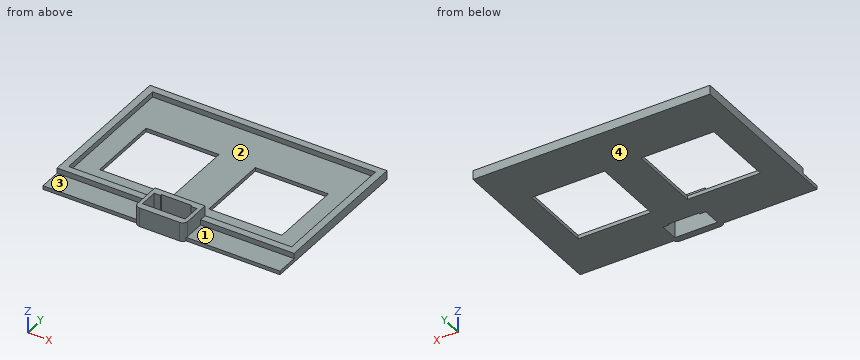
```python
from build123d import *

# Parameters (mm, degrees)
F0_W     = 38.1
F0_H     = 38.1
F1_DEPTH = 1.905
F0_W_2   = 48.74895
F0_H_2   = 11.557
F0_W_3   = 48.79975
F2_DEPTH = 4.699
F0_W_4   = 13.589
F0_H_3   = 3.5052
F3_DEPTH = 9.9314
F4_R     = 2.54


# Not quite as in the source:
# - a feature names something its author has since deleted; it is built from what else it names


with BuildPart() as f1:
    # F0 (on Top) → F1 (new body)
    with BuildSketch(Plane.XY):
        Polygon((-13.10005, -34.417), (13.04925, -34.417), (58.166, -34.417), (58.166, 34.417), (-58.166, 34.417), (-58.166, -34.417), align=None)
        with Locations((-28.5115, -6.604)):
            Rectangle(F0_W, F0_H, mode=Mode.SUBTRACT)
        with Locations((28.5115, -6.604)):
            Rectangle(F0_W, F0_H, mode=Mode.SUBTRACT)
    extrude(amount=F1_DEPTH)



with BuildPart() as f1b:
    # F0 (on Top) → F1, piece 2 (new body)
    with BuildSketch(Plane.XY):
        with Locations((-37.474525, -43.8785)):
            Rectangle(F0_W_2, F0_H_2)
    extrude(amount=F1_DEPTH)


with BuildPart() as f1c:
    # F0 (on Top) → F1, piece 3 (new body)
    with BuildSketch(Plane.XY):
        with Locations((37.449125, -43.8785)):
            Rectangle(F0_W_3, F0_H_2)
    extrude(amount=F1_DEPTH)


with BuildPart() as f1_1:
    add(f1.part)

    add(f1b.part)  # F2 merges F1b

    add(f1c.part)  # F2 merges F1c
    # F0 (on Top) → F2 (join)
    with BuildSketch(Plane.XY):
        Polygon((61.849, -38.1), (61.849, 38.1), (-61.849, 38.1), (-61.849, -38.1), (-13.10005, -38.1), (-13.10005, -34.417), (-58.166, -34.417), (-58.166, 34.417), (58.166, 34.417), (58.166, -34.417), (13.04925, -34.417), (13.04925, -38.1), align=None)
    extrude(amount=F2_DEPTH)

    # F0 (on Top) → F3 (join)
    with BuildSketch(Plane.XY):
        Polygon((11.14425, -38.1), (13.04925, -38.1), (13.04925, -34.417), (-13.10005, -34.417), (-13.10005, -38.1), (-11.14425, -38.1), (-8.001, -38.1), (-8.001, -37.2745), (8.001, -37.2745), (8.001, -38.1), align=None)
        Polygon((-11.14425, -38.1), (-13.10005, -38.1), (-13.10005, -49.657), (-13.10005, -51.2572), (-6.7945, -51.2572), (-6.7945, -47.752), (-11.14425, -47.752), align=None)
        Polygon((13.04925, -49.657), (13.04925, -38.1), (11.14425, -38.1), (11.14425, -47.752), (6.7945, -47.752), (6.7945, -51.2572), (13.04925, -51.2572), align=None)
        with Locations((0, -49.5046)):
            Rectangle(F0_W_4, F0_H_3)
    extrude(amount=F3_DEPTH)

    # F4
    f4_edges = [f1_1.edges().sort_by_distance(p)[0] for p in [
        (-13.10005, -51.2572, 4.9657),
        (13.04925, -51.2572, 4.9657),
    ]]
    fillet(f4_edges, radius=F4_R)


solid = f1_1.part
```
Check sheet for the modelled part. Datum: model origin and axes. Units: mm. Face numbers are marked on the shaded views. A direction names the side the tool comes from. Round coordinates to 2 decimals unless told otherwise and drop trailing zeros. Order: outer loops, then holes, each group sorted by start corner. A loop starts at its lowest first (then second) coordinate and runs counter-clockwise, first axis right, second up. Notation, with made-up numbers: (11, -29.75) - (57, -29.75) arc R21 cw to (57, -0.75) - close; hole circle Ø1 at (-12.5, -32.75). An arc over 180 degrees is marked (long way). Write item = value, one per line.
Q1. Section check A-A (y = -14). Record the boundary of the cut face in (x, z) (1 decimal), and give its area (3 significant figures).
Computed:
outline = (-61.8, 0) - (-47.6, 0) - (-47.6, 1.9) - (-58.2, 1.9) - (-58.2, 4.7) - (-61.8, 4.7) - close; (-9.5, 0) - (9.5, 0) - (9.5, 1.9) - (-9.5, 1.9) - close; (47.6, 0) - (61.8, 0) - (61.8, 4.7) - (58.2, 4.7) - (58.2, 1.9) - (47.6, 1.9) - close
area = 111 mm^2
Q2. Thickness scan on line 1 along Y through (x, z) = (6, 2.25); line 2 along X through (y, z) = (-22.5, 3.25); line 3 along X through (y, z) = (-38, 5.5). Record the ranges inside material, lowest first.
Computed:
line_1 = -51.26 to -47.75, -37.27 to -34.42, 34.42 to 38.1
line_2 = -61.85 to -58.17, 58.17 to 61.85
line_3 = -13.1 to -8, 8 to 13.05
Q3. Tool access check on the marked faces 3 and 4. Record the directions out of +Z, -Z, +X, -X, +Y, -Y that give a thin tool (end or side, any length) a straight path to the whole face; none if there is none.
Computed:
face_3 = +Z, -X, -Y
face_4 = -Z, +X, -X, +Y, -Y
Q4. Section check B-B (x = -3). Record the boundary of the cut face in (y, z) (1 decimal).
Computed:
outline = (-51.3, 0) - (-47.8, 0) - (-47.8, 9.9) - (-51.3, 9.9) - close; (-37.3, 0) - (38.1, 0) - (38.1, 4.7) - (34.4, 4.7) - (34.4, 1.9) - (-34.4, 1.9) - (-34.4, 9.9) - (-37.3, 9.9) - close
Q5. Go/stop test with flat-tipped pins: pin 1 (23 mm diameter, centred on x = 0, y = 10.5, fed in from +Z) (3 decimals); pin 2 (1 mm diameter, centred on x = 32, z = 1, fed in from -Y); pin 3 (2 mm diameter, centred on x = -28, z = 4, fed in from -Y). Record where each tip stops, or that it passes through.
Computed:
pin_1 = 1.905
pin_2 = -49.66
pin_3 = -38.1
Q6. Draft check along X on the marked faces 1 and 2. Enter one of: pulls with the +X half, pulls with the -X half, needs draft (parallel to the pull), parting line crosses it, or undercut.
Computed:
face_1 = needs draft
face_2 = undercut
Q7. Section check C-C (y = 21). Record the boundary of the cut face in (x, z) (3 decimals).
Computed:
outline = (-61.849, 0) - (61.849, 0) - (61.849, 4.699) - (58.166, 4.699) - (58.166, 1.905) - (-58.166, 1.905) - (-58.166, 4.699) - (-61.849, 4.699) - close
Q8. Section check D-D (x = 53.5). Record the boundary of the cut face in (y, z) (3 decimals), and give its area (3 significant figures).
Computed:
outline = (-49.657, 0) - (38.1, 0) - (38.1, 4.699) - (34.417, 4.699) - (34.417, 1.905) - (-34.417, 1.905) - (-34.417, 4.699) - (-38.1, 4.699) - (-38.1, 1.905) - (-49.657, 1.905) - close
area = 188 mm^2
